Autodesk Inventor part; units mm, degrees
ref_plane "YZ Plane" through (0, 0, 0) normal (1, 0, 0) x (0, 1, 0)
ref_plane "XZ Plane" through (0, 0, 0) normal (0, 1, 0) x (-1, 0, 0)
ref_plane "XY Plane" through (0, 0, 0) normal (0, 0, 1) x (1, 0, 0)
sketch "Sketch1" plane through (0, 0, 0) normal (0, 0, 1) x (1, 0, 0)
  line L0 (-4.8, 0) -> (0.8, 0) construction
  line L1 (-3.15, 0) -> (-3.15, 9)
  line L2 (-3.15, 9) -> (-4, 9)
  line L3 (-4, 9) -> (-4, 49)
  line L4 (-4, 49) -> (-3, 55)
  line L5 (-3, 55) -> (-3, 80)
  line L6 (-3, 80) -> (-4, 80)
  line L7 (-4, 80) -> (-4, 88.25)
  line L8 (-4, 88.25) -> (-3.8469, 90)
  line L9 (-3.8469, 90) -> (-2, 90)
  line L10 (-2, 90) -> (0, 92)
  line L11 (0, 92) -> (0, 0)
  line L12 (-3.15, 0) -> (0, 0)
  dimension "d1" = 92
  dimension "d16" = 45
  dimension "d18" = 3.75
  dimension "d19" = 12
  dimension "d20" = 37
  dimension "d21" = 43
  dimension "d22" = 5
  dimension "d23" = 2
  dimension "d29" = 9
  dimension "d31" = 6.3
  dimension "d32" = 8
  dimension "d33" = 6
  dimension "d34" = 8
revolve "Revolution3" add sketch "Sketch1" angle 360 about axis through (0, 92, 0) along (0, -1, 0)
properties part number "DORMER_SPU4908_M8SpiralFl_TAP"
Verification items for the finished model (mm, model axes). A direction names the side the tool comes from. Give positions to 0.01 mm unless a question says otherwise; leave off trailing zeros. Loops run counter-clockwise (first coordinate to the right, second up) from the corner with the lowest first, then second, coordinate; pieces in that order, holes last. Notation, with made-up numbers: M 47.25,-31.75 L 76.25,-31.75 A18 cw 76.25,-27.75 Z; hole C 54,76.5 d1. An arc over 180 degrees is marked long. One line per question, with ' | ' between items.
Item 1: Thickness scan on line 1 (Y direction, x = -2.75, z = -0.75); line 2 (X direction, y = 40, z = -0.25); line 3 (Z direction, x = -1.75, y = 65). Record the ranges inside material, lowest first. Write a range as [from, to].
Completed:
line 1: y = [0, 90] | line 2: x = [-3.99, 3.99] | line 3: z = [-2.44, 2.44]
Item 2: Draft check along Y on faces 1 (the face through (-3.24, 52.62, -1.02)), 2 (the face through (0, 0, 0)), 3 (the face through (-1, 80, -3)), 4 (the face through (0.867, 84.183, -3.905)). Enter one of: +Y half, -Y half, draft (parallel to the pull), parting line (faces both ways), or undercut.
Completed:
face 1: undercut | face 2: -Y half | face 3: undercut | face 4: draft
Item 3: Section check A-A, the plane y = 66. Record the cut outline in (x, z).
Completed:
outline: C 0,0 d6
Item 4: Section check B-B, the plane y = 44.5. Record the cut outline in (x, z), plus the area to 3 significant figures.
Completed:
outline: C 0,0 d8 | area: 50.3 mm^2
Item 5: Depth check by flat-ended pin: P1, Ø1.5, axis at x = -2.5, y = 60, coming from the +Z side; P2, Ø1, axis at x = -3, y = 42.5, coming from the -Z side. Enter the tip coordinate at first touch or a pass-through.
Completed:
P1: stops at z = 2.44 | P2: stops at z = -3.12
Item 6: Tool access check on faces 5 (the face through (2.5, 4.563, -1.917)), 6 (the face through (0.867, 29.28, -3.905)), 7 (the face through (3, 68, 0)), 8 (the face through (-2, 90, 2)). Record the directions out of +Z, -Z, +X, -X, +Y, -Y that give a thin tool (end or side, any length) a straight path to the whole face; none if there is none.
Completed:
face 5: -Y | face 6: +Y, -Y | face 7: none | face 8: +Y
